Part model, mm, in its own coordinate system. Face numbers are marked on the shaded views. A direction names the side the tool comes from. Round coordinates to 2 decimals unless told otherwise and drop trailing zeros. Loops run counter-clockwise (first coordinate to the right, second up) from the corner with the lowest first, then second, coordinate; pieces in that order, holes last. Notation, with made-up numbers: M 20,46 L 54,46 A19 cw 54,81 Z; hole C 22.25,77.5 d1. An arc over 180 degrees is marked long. Put each result on its own line as item: value. Start each with the question number.
1) Slice it at C-C on x = 17. Give the cut face in (y, z), then the cut area to 3 significant figures.
2) Drop flat-ended pins along their axis: pin 1 Ø1 at (x, y) = (13, -3.5) entering from -Z; pin 2 Ø4.5 at (x, z) = (15, 0) entering from +Y; pin 3 Ø1 at (y, z) = (-1.5, -6.5) entering from -X; pin 4 Ø1 at (x, y) = (-0.5, -1.5) entering from +Z. Give the stop position or say it passes through.
3) Which spindle directions (+Z, -Z, +X, -X, +Y, -Y) get a long thin tool onto all of the face, cutting with end or side? Do the marked faces 5 and 6. Say none if no direction does.
4) Pull direction X, two halves, no side cores. Call the marked faces 1, 2, 3 and 4: +X half, -X half, draft (parallel to the pull), parting line (faces both ways), or undercut.
5) Slice it at A-A on z = 0. Give the cut face in (x, y), then the cut area to 3 significant figures.
6) Slice it at D-D on y = -5. Give the cut face in (x, z).
7) Probe line 1 along X through (y, z) = (-1.5, -0.75); line 2 along X through (y, z) = (-5, 1.25); line 3 along Z through (x, y) = (15, -3.75). List the from-to ranges inside material, lowest first.
8) Slice it at B-B on z = -3. Give the cut face in (x, y), then the cut area to 3 significant figures.
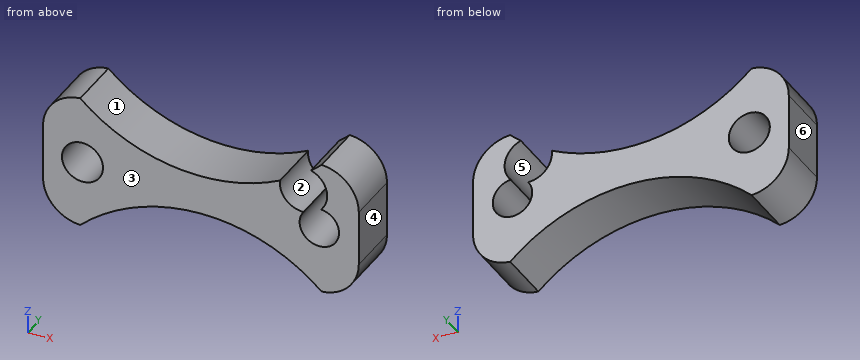
```python
from build123d import *

# Parameters (mm, degrees)
F1_DEPTH = 7
F3_D     = 5.2
F5_D     = 5
F7_D     = 45
F9_D     = 45
F11_D    = 6


with BuildPart() as f1:
    # F0 (on Front) → F1 (new body)
    with BuildSketch(Plane.XZ):
        with BuildLine():
            Line((-15, -8.5), (15, -8.5))
            ThreePointArc((15, -8.5), (18.5355339059, -7.0355339059), (20, -3.5))
            Line((20, -3.5), (20, 3.5))
            ThreePointArc((20, 3.5), (18.5355339059, 7.0355339059), (15, 8.5))
            Line((15, 8.5), (-15, 8.5))
            ThreePointArc((-15, 8.5), (-18.5355339059, 7.0355339059), (-20, 3.5))
            Line((-20, 3.5), (-20, -3.5))
            ThreePointArc((-20, -3.5), (-18.5355339059, -7.0355339059), (-15, -8.5))
        make_face()
    extrude(amount=F1_DEPTH)

    # F3 (through all)
    with Locations(Plane(origin=(0, 0, 0), x_dir=(1, 0, 0), z_dir=(0, 1, 0))):
        with Locations((-15, 0)):
            Hole(F3_D / 2)

    # F5 (through all)
    with Locations(Plane(origin=(0, 0, 0), x_dir=(1, 0, 0), z_dir=(0, 1, 0))):
        with Locations((15, 0)):
            Hole(F5_D / 2)

    # F7 (through all)
    with Locations(Plane(origin=(0, 0, 0), x_dir=(1, 0, 0), z_dir=(0, 1, 0))):
        with Locations((0, 25)):
            Hole(F7_D / 2)

    # F9 (through all)
    with Locations(Plane(origin=(0, 0, 0), x_dir=(1, 0, 0), z_dir=(0, 1, 0))):
        with Locations((0, -25)):
            Hole(F9_D / 2)

    # F11 (through all)
    with Locations(Plane(origin=(0, 0, 0), x_dir=(1, 0, 0), z_dir=(0, 1, 0))):
        with Locations((13, -4.5)):
            Hole(F11_D / 2)


solid = f1.part
```
Recorded:
1. outline: M -7,-8.08 L 0,-8.08 L 0,-1.5 L -7,-1.5 Z; M -7,1.5 L 0,1.5 L 0,8.08 L -7,8.08 Z
1. area: 92.2 mm2
2. pin 1: stops at z = -7
2. pin 2: passes through
2. pin 3: stops at x = -19.33
2. pin 4: stops at z = 2.52
3. face 5: +Y, -Y
3. face 6: +Z, -Z, -X, +Y, -Y
4. face 1: undercut
4. face 2: undercut
4. face 3: draft
4. face 4: +X half
5. outline: M -20,-7 L -17.6,-7 L -17.6,0 L -20,0 Z; M -12.4,-7 L 12.5,-7 L 12.5,0 L -12.4,0 Z; M 17.5,-7 L 20,-7 L 20,0 L 17.5,0 Z
5. area: 209 mm2
6. outline: M -20,-3.5 A5 ccw -15.29,-8.49 A22.5 cw 15.29,-8.49 A5 ccw 20,-3.5 L 20,3.5 A5 ccw 15.29,8.49 A22.5 cw 13.95,7.35 A3 cw 15.23,2.49 A2.5 cw long 13,1.5 A3 cw 10.02,4.85 A22.5 cw -15.29,8.49 A5 ccw -20,3.5 Z; hole C -15,0 d5.2
7. line 1: x = -20 to -17.49, -12.51 to 12.62, 17.38 to 20
7. line 2: x = -20 to -17.28, -12.72 to 12.83, 17.17 to 20
7. line 3: z = -8.23 to -2.5, 6.74 to 8.23
8. outline: M -20,-7 L -4.72,-7 L -4.72,0 L -20,0 Z; M 4.72,-7 L 20,-7 L 20,0 L 4.72,0 Z
8. area: 214 mm2
